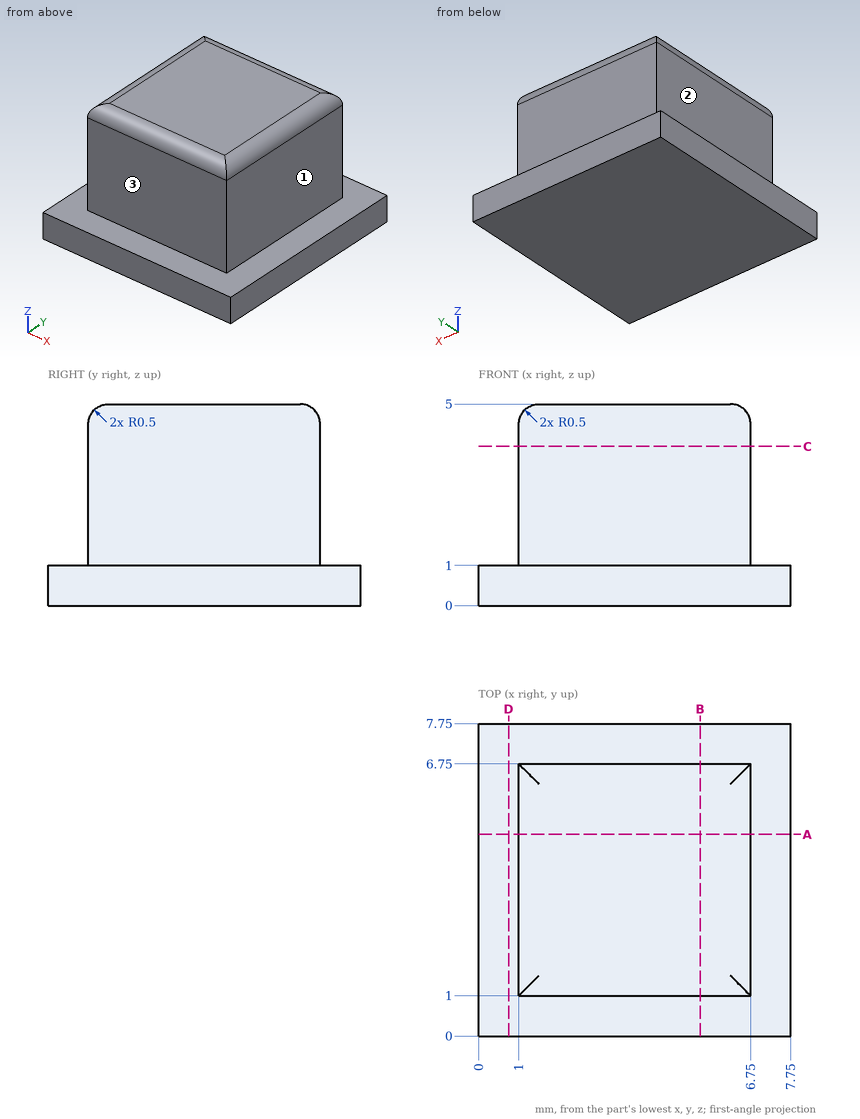
The drawing under review shows one solid part. Ordinate dimensions are in mm from its lowest x, y, z. A direction names the side the tool comes from. Give positions to 0.01 mm unless a question says otherwise; leave off trailing zeros. Loops run counter-clockwise (first coordinate to the right, second up) from the corner with the lowest first, then second, coordinate; pieces in that order, holes last. Notation, with made-up numbers: M -15,46.25 L 13,46.25 A27 ccw 13,70.25 Z; hole C 28.25,68 d6. An arc over 180 degrees is marked long. One line per item, written item: value. Start each with the question number.
Q1. For L1, parallel to X at y = 2, z = 3.55; L2, parallel to Z at x = 7.25, y = 6, list the stretches that pass through material, from the lowest coordinate up.
Q2. Add section A-A (y = 5). Give the boundary of the cut face in (x, z).
Q3. Add section C-C (z = 3.95). Give the boundary of the cut face in (x, y).
Q4. Add section D-D (x = 0.75). Give the boundary of the cut face in (y, z).
Q5. Machinability: for the marked faces 1, 2 and 3, which of the approach directions +Z, -Z, +X, -X, +Y, -Y give a long, thin tool a straight path to every point of the face, cutting with its end or side? Answer none if there is none.
Q6. Clearance check with flat-ended pins moving along their axes: pin 1 Ø2 at (y, z) = (1, 4.5) entering from -X; pin 2 Ø2 at (x, z) = (7, 2.5) entering from +Y. State where each tip first meets the part, or that it passes through.
Reply:
1. L1: 1 to 6.75
1. L2: 0 to 1
2. outline: M 0,0 L 7.75,0 L 7.75,1 L 6.75,1 L 6.75,4.5 A0.5 ccw 6.25,5 L 1.5,5 A0.5 ccw 1,4.5 L 1,1 L 0,1 Z
3. outline: M 1,1 L 6.75,1 L 6.75,6.75 L 1,6.75 Z
4. outline: M 0,0 L 7.75,0 L 7.75,1 L 0,1 Z
5. face 1: +Z, +X, +Y, -Y
5. face 2: +Z, -X, +Y, -Y
5. face 3: +Z, +X, -X, -Y
6. pin 1: x = 1
6. pin 2: y = 6.75
